Design review of the part built by this model. Coordinates are the model's own, in mm. A direction names the side the tool comes from. Give positions to 0.01 mm unless a question says otherwise; leave off trailing zeros. Write each loop counter-clockwise with the first axis right and the second up, starting at its lowest first coordinate (ties: lowest second). Pieces come first, ordered by that corner, then holes.
```python
from build123d import *

# Parameters (mm, degrees)
SKETCH1_W           = 48.2092
SKETCH1_H           = 40.5892
BOSS_EXTRUDE1_DEPTH = 12.7
SHELL1_T            = -2
CUT_EXTRUDE2_DEPTH  = 68.58
FILLET6_R           = 2.54
FILLET7_R           = 2.54
FILLET8_R           = 2.54
FILLET9_R           = 2.54
FILLET10_R          = 2.54
SKETCH6_W           = 39.1292
SKETCH6_H           = 31.5092
CUT_EXTRUDE4_DEPTH  = 68.58
CUT_EXTRUDE5_DEPTH  = 49.276
FILLET19_R          = 3.0988


with BuildPart() as part:
    # Sketch1 → Boss-Extrude1 (new body)
    with BuildSketch(Plane(origin=(0, 0, 0), x_dir=(1, 0, 0), z_dir=(0, 1, 0))):
        Rectangle(SKETCH1_W, SKETCH1_H)
    extrude(amount=BOSS_EXTRUDE1_DEPTH)

    # Shell1
    shell1_openings = [part.faces().sort_by_distance(p)[0] for p in [
        (0, 0, 0),
    ]]
    offset(amount=SHELL1_T, openings=shell1_openings, kind=Kind.INTERSECTION)

    # Sketch4 → Cut-Extrude2 (cut)
    with BuildSketch(Plane.ZY.offset(24.1046)):
        Polygon((0, 0), (6.35, 0), (6.35, 10.69848), (-6.3246, 10.69848), (-6.3246, 0), align=None)
    extrude(amount=-CUT_EXTRUDE2_DEPTH, mode=Mode.SUBTRACT)

    # Fillet6
    # the kernel refuses this fillet: 2.54 mm, written as the material it takes off along each edge
    with BuildSketch(Plane(origin=(30.4546, 12.7, -20.2946), x_dir=(0, -1, 0), z_dir=(-1, 0, 0))) as fillet6_piece_1:
        with BuildLine():
            CenterArc((FILLET6_R, FILLET6_R), FILLET6_R, 180, 90)
            Line((0, FILLET6_R), (0, 0))
            Line((0, 0), (FILLET6_R, 0))
        make_face()
    extrude(amount=60.9092, mode=Mode.SUBTRACT)
    with BuildSketch(Plane(origin=(24.1046, 12.7, 26.6446), x_dir=(0, -1, 0), z_dir=(0, 0, -1)), Plane(origin=(-24.1046, 12.7, -26.6446), x_dir=(0, -1, 0), z_dir=(0, 0, 1))) as fillet6_piece_2:
        with BuildLine():
            CenterArc((FILLET6_R, FILLET6_R), FILLET6_R, 180, 90)
            Line((0, FILLET6_R), (0, 0))
            Line((0, 0), (FILLET6_R, 0))
        make_face()
    extrude(amount=53.2892, mode=Mode.SUBTRACT)
    with BuildSketch(Plane(origin=(-30.4546, 12.7, 20.2946), x_dir=(0, 0, -1), z_dir=(1, 0, 0))) as fillet6_piece_3:
        with BuildLine():
            CenterArc((FILLET6_R, -FILLET6_R), FILLET6_R, 90, 90)
            Line((0, -FILLET6_R), (0, 0))
            Line((0, 0), (FILLET6_R, 0))
        make_face()
    extrude(amount=60.9092, mode=Mode.SUBTRACT)

    # Fillet7
    # the kernel refuses this fillet: 2.54 mm, written as the material it takes off along each edge
    with BuildSketch(Plane(origin=(-21.5646, 10.16, -17.7546), x_dir=(-1, 0, 0), z_dir=(0, 0, -1))) as fillet7_piece_1_section:
        Polygon((0, 0), (FILLET7_R, 0), (FILLET7_R, FILLET7_R), (0, FILLET7_R), align=None)
    fillet7_piece_1 = extrude(amount=FILLET7_R, mode=Mode.PRIVATE)
    fillet7_piece_1 = fillet7_piece_1 - Plane(origin=(-21.5646, 10.16, -17.7546), x_dir=(0.7071067811865475, -0.7071067811865475, 0), z_dir=(0, 0, -1)) * Sphere(FILLET7_R, mode=Mode.PRIVATE)
    add(fillet7_piece_1, mode=Mode.SUBTRACT)
    with BuildSketch(Plane(origin=(-24.1046, -6.35, -20.2946), x_dir=(1, 0, 0), z_dir=(0, 1, 0))) as fillet7_piece_2:
        with BuildLine():
            CenterArc((FILLET7_R, -FILLET7_R), FILLET7_R, 90, 90)
            Line((0, -FILLET7_R), (0, 0))
            Line((0, 0), (FILLET7_R, 0))
        make_face()
    extrude(amount=16.51, mode=Mode.SUBTRACT)

    # Fillet8
    # the kernel refuses this fillet: 2.54 mm, written as the material it takes off along each edge
    with BuildSketch(Plane(origin=(-21.5646, 10.16, 17.7546), x_dir=(-1, 0, 0), z_dir=(0, 0, 1))) as fillet8_piece_1_section:
        Polygon((0, 0), (FILLET8_R, 0), (FILLET8_R, -FILLET8_R), (0, -FILLET8_R), align=None)
    fillet8_piece_1 = extrude(amount=FILLET8_R, mode=Mode.PRIVATE)
    fillet8_piece_1 = fillet8_piece_1 - Plane(origin=(-21.5646, 10.16, 17.7546), x_dir=(0.7071067811865475, -0.7071067811865475, 0), z_dir=(0, 0, 1)) * Sphere(FILLET8_R, mode=Mode.PRIVATE)
    add(fillet8_piece_1, mode=Mode.SUBTRACT)
    with BuildSketch(Plane(origin=(-24.1046, -6.35, 20.2946), x_dir=(1, 0, 0), z_dir=(0, 1, 0))) as fillet8_piece_2:
        with BuildLine():
            CenterArc((FILLET8_R, FILLET8_R), FILLET8_R, 180, 90)
            Line((0, FILLET8_R), (0, 0))
            Line((0, 0), (FILLET8_R, 0))
        make_face()
    extrude(amount=16.51, mode=Mode.SUBTRACT)

    # Fillet9
    # the kernel refuses this fillet: 2.54 mm, written as the material it takes off along each edge
    with BuildSketch(Plane(origin=(21.5646, 10.16, -17.7546), x_dir=(1, 0, 0), z_dir=(0, 0, -1))) as fillet9_piece_1_section:
        Polygon((0, 0), (FILLET9_R, 0), (FILLET9_R, -FILLET9_R), (0, -FILLET9_R), align=None)
    fillet9_piece_1 = extrude(amount=FILLET9_R, mode=Mode.PRIVATE)
    fillet9_piece_1 = fillet9_piece_1 - Plane(origin=(21.5646, 10.16, -17.7546), x_dir=(-0.7071067811865475, -0.7071067811865475, 0), z_dir=(0, 0, -1)) * Sphere(FILLET9_R, mode=Mode.PRIVATE)
    add(fillet9_piece_1, mode=Mode.SUBTRACT)
    with BuildSketch(Plane(origin=(24.1046, -6.35, -20.2946), x_dir=(-1, 0, 0), z_dir=(0, 1, 0))) as fillet9_piece_2:
        with BuildLine():
            CenterArc((FILLET9_R, FILLET9_R), FILLET9_R, 180, 90)
            Line((0, FILLET9_R), (0, 0))
            Line((0, 0), (FILLET9_R, 0))
        make_face()
    extrude(amount=16.51, mode=Mode.SUBTRACT)

    # Fillet10
    # the kernel refuses this fillet: 2.54 mm, written as the material it takes off along each edge
    with BuildSketch(Plane(origin=(21.5646, 10.16, 17.7546), x_dir=(1, 0, 0), z_dir=(0, 0, 1))) as fillet10_piece_1_section:
        Polygon((0, 0), (FILLET10_R, 0), (FILLET10_R, FILLET10_R), (0, FILLET10_R), align=None)
    fillet10_piece_1 = extrude(amount=FILLET10_R, mode=Mode.PRIVATE)
    fillet10_piece_1 = fillet10_piece_1 - Plane(origin=(21.5646, 10.16, 17.7546), x_dir=(-0.7071067811865475, -0.7071067811865475, 0), z_dir=(0, 0, 1)) * Sphere(FILLET10_R, mode=Mode.PRIVATE)
    add(fillet10_piece_1, mode=Mode.SUBTRACT)
    with BuildSketch(Plane(origin=(24.1046, -6.35, 20.2946), x_dir=(-1, 0, 0), z_dir=(0, 1, 0))) as fillet10_piece_2:
        with BuildLine():
            CenterArc((FILLET10_R, -FILLET10_R), FILLET10_R, 90, 90)
            Line((0, -FILLET10_R), (0, 0))
            Line((0, 0), (FILLET10_R, 0))
        make_face()
    extrude(amount=16.51, mode=Mode.SUBTRACT)

    # Sketch6 → Cut-Extrude4 (cut)
    with BuildSketch(Plane(origin=(0, 12.7, 0), x_dir=(1, 0, 0), z_dir=(0, 1, 0))):
        Rectangle(SKETCH6_W, SKETCH6_H)
    extrude(amount=-CUT_EXTRUDE4_DEPTH, mode=Mode.SUBTRACT)

    # Sketch3 → Cut-Extrude5 (cut)
    with BuildSketch(Plane.XY.offset(20.2946)):
        Polygon((14.4526, 10.69848), (-12.1666, 10.69848), (-14.7066, 10.69848), (-14.7066, 0), (14.4526, 0), align=None)
    extrude(amount=-CUT_EXTRUDE5_DEPTH, mode=Mode.SUBTRACT)

    # Fillet19
    fillet19_edges = [part.edges().sort_by_distance(p)[0] for p in [
        (-22.1046, 5.35, -18.2946),
        (-22.1046, 5.35, 18.2946),
        (22.1046, 5.35, 18.2946),
        (22.1046, 5.35, -18.2946),
    ]]
    fillet(fillet19_edges, radius=FILLET19_R)


solid = part.part
```
(1) Consider section A-A, the plane y = 7. Give the number of separate pieces and of enclosed holes in the cut face, then the cut area to 3 significant figures.
Resolved:
separate pieces: 4
enclosed holes: 0
area: 175 mm2
(2) To check wall thickness, follow L1, parallel to X at y = 6, z = -7.5; L2, parallel to Z at x = 17, y = 7; L3, parallel to Y at x = -1.5, z = -18. State the ranges of each line that lie inside material, in increasing order.
Resolved:
L1: x = -24.1 to -22.1, 22.1 to 24.1
L2: z = -20.29 to -18.29, 18.29 to 20.29
L3: y = 10.7 to 12.69
(3) Consider section D-D, the plane x = -16. Give the boundary of the cut face in (y, z), then the cut area to 3 significant figures.
Resolved:
outline: (0, -20.29) - (10.16, -20.29) arc R2.54 ccw to (12.7, -17.75) - (12.7, -15.75) - (10.7, -15.75) - (10.7, -18.29) - (0, -18.29) - close; (0, 18.29) - (10.7, 18.29) - (10.7, 15.75) - (12.7, 15.75) - (12.7, 17.75) arc R2.54 ccw to (10.16, 20.29) - (0, 20.29) - close
area: 58.2 mm2
(4) Clearance check with flat-ended pins moving along their axes: P1, Ø1.6, axis at x = -3, y = 12, coming from the -Z side; P2, Ø0.6, axis at y = 4, z = 19.5, coming from the +X side; P3, Ø1.6, axis at y = 4, z = -19, coming from the -X side; P4, Ø6, axis at x = -3, z = 13, coming from the +Y side. State where each tip first meets the part, or that it passes through.
Resolved:
P1: stops at z = -20.07
P2: stops at x = 23.65
P3: stops at x = -24.07
P4: stops at y = 12.7
(5) Mouldability with a two-part tool opening along Z and no side actions: class faces 1 (the face through (-23, 0, -15)), 2 (the face through (21.173, 5.425, 17.411)), 3 (the face through (0.302, 11.976, -19.531)), 4 (the face through (0, 12, -15.755)) as pulls with the +Z half, pulls with the -Z half, needs draft (parallel to the pull), parting line crosses it, or undercut.
Resolved:
face 1: needs draft
face 2: undercut
face 3: pulls with the -Z half
face 4: undercut
(6) Tool access review of faces 5 (the face through (23, 5, -6.325)), 6 (the face through (0, 10.698, -19)), 7 (the face through (-21.221, 5.275, 17.363)), 8 (the face through (22.5, 0, 15.9)), 9 (the face through (19.565, 12, 0)): name each direction out of +Z, -Z, +X, -X, +Y, -Y from which nothing blocks a thin tool from reaching the whole face with its end or side.
Resolved:
face 5: +X, -X, -Y
face 6: +Z, -Z, -Y
face 7: -Y
face 8: +Z, -Z, +X, -X, -Y
face 9: +Y, -Y
